Drawing for the job (mm, zero at the part's lowest x, y, z). A direction names the side the tool comes from. Give positions to 0.01 mm unless a question says otherwise; leave off trailing zeros. Order: outer loops, then holes, each group sorted by start corner. A loop starts at its lowest first (then second) coordinate and runs counter-clockwise, first axis right, second up. Notation, with made-up numbers: (20.5, 59.25) - (24.5, 59.25) arc R14 cw to (24.5, 73.25) - close; hole circle Ø9 at (-27, 19). An arc over 180 degrees is marked (long way). Use CSV: the item, a comma, the result in double quotes. Start each with the question number.
(1) Band-saw the part on A-A, the plane z = 7.62. Give the cut face in (x, y).
(2) Band-saw the part on C-C, the plane y = 10.5. Give the cut face in (x, z) (3 decimals), then the cut area to 3 significant figures.
(3) Pull direction X, two halves, no side cores. Call the marked faces 1, 2 and 3: +X half, -X half, draft (parallel to the pull), parting line (faces both ways), or undercut.
(4) Band-saw the part on B-B, the plane x = 11.27. Give the cut face in (y, z).
(5) Drop flat-ended pins along their axis: pin 1 Ø4 at (y, z) = (9, 10.5) entering from +X; pin 2 Ø5 at (x, y) = (24.5, 5.5) entering from -Z; pin 3 Ø6.5 at (y, z) = (3.5, 7) entering from -X; pin 4 Ø3 at (x, z) = (19.5, 5.5) entering from -Y. Give the stop position or say it passes through.
(6) Band-saw the part on D-D, the plane x = 5. Give the cut face in (y, z).
(7) Tool access for the marked faces 4, 5, 6 and 7: list every direction of +Z, -Z, +X, -X, +Y, -Y with a clear straight run to the whole face (end or side of a thin tool).
(8) Probe L1, parallel to Z at x = 5.5, y = 12.25; L2, parallel to X at y = 5, z = 7.62; L3, parallel to X at y = 2.5, z = 8.5. List the from-to ranges inside material, lowest first.
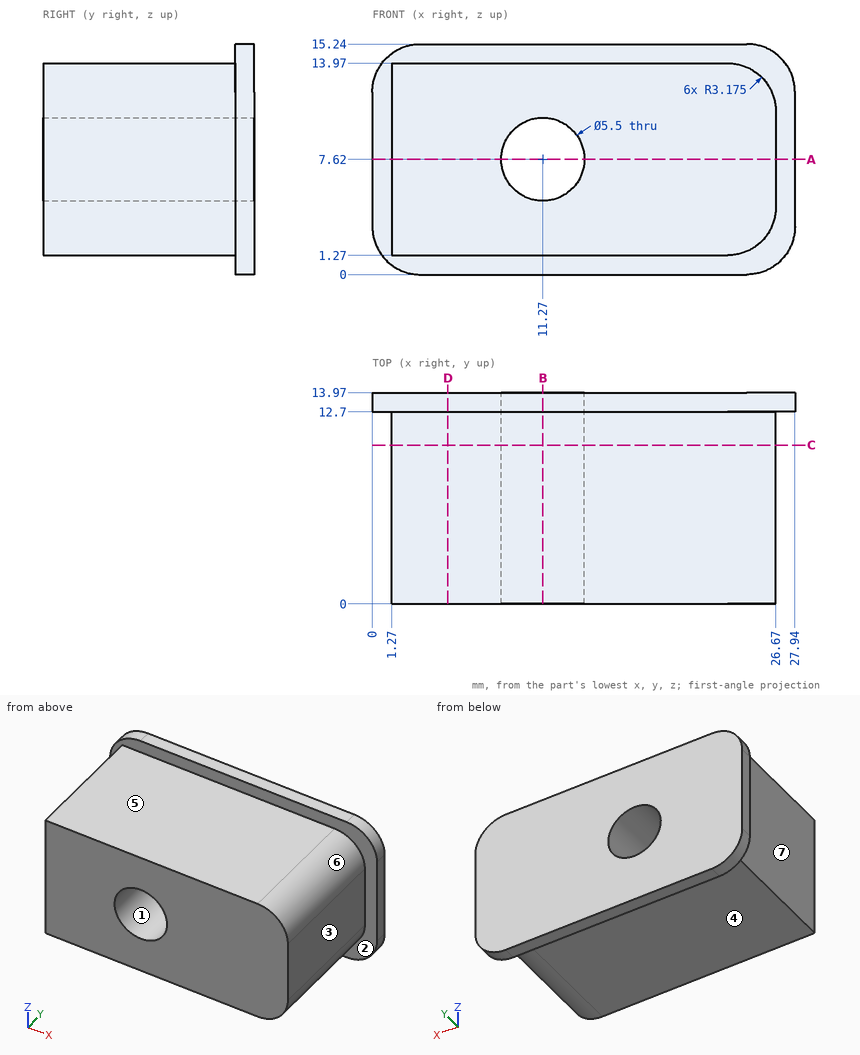
Answer block:
1,outline,"(0, 12.7) - (1.27, 12.7) - (1.27, 0) - (8.52, 0) - (8.52, 13.97) - (0, 13.97) - close; (14.02, 0) - (26.67, 0) - (26.67, 12.7) - (27.94, 12.7) - (27.94, 13.97) - (14.02, 13.97) - close"
2,outline,"(1.27, 1.27) - (23.495, 1.27) arc R3.175 ccw to (26.67, 4.445) - (26.67, 10.795) arc R3.175 ccw to (23.495, 13.97) - (1.27, 13.97) - close; hole circle Ø5.5 at (11.27, 7.62)"
2,area,"294 mm2"
3,face 1,"undercut"
3,face 2,"draft"
3,face 3,"+X half"
4,outline,"(0, 1.27) - (12.7, 1.27) - (12.7, 0) - (13.97, 0) - (13.97, 4.87) - (0, 4.87) - close; (0, 10.37) - (13.97, 10.37) - (13.97, 15.24) - (12.7, 15.24) - (12.7, 13.97) - (0, 13.97) - close"
5,pin 1,"stops at x = 26.67"
5,pin 2,"stops at z = 1.27"
5,pin 3,"stops at x = 1.27"
5,pin 4,"stops at y = 0"
6,outline,"(0, 1.27) - (12.7, 1.27) - (12.7, 0) - (13.97, 0) - (13.97, 15.24) - (12.7, 15.24) - (12.7, 13.97) - (0, 13.97) - close"
7,face 4,"-Z, +X, -X, -Y"
7,face 5,"+Z, +X, -X, -Y"
7,face 6,"+Z, +X, -Y"
7,face 7,"+Z, -Z, -X, -Y"
8,L1,"z = 1.27 to 13.97"
8,L2,"x = 1.27 to 8.52, 14.02 to 26.67"
8,L3,"x = 1.27 to 8.66, 13.88 to 26.67"
